For this review, take the finished solid that the model builds, in its own axes (mm). Face numbers are marked on the shaded views. A direction names the side the tool comes from. Give positions to 0.01 mm unless a question says otherwise; leave off trailing zeros. Write each loop counter-clockwise with the first axis right and the second up, starting at its lowest first coordinate (ties: lowest second). Pieces come first, ordered by that corner, then holes. Notation, with made-up numbers: (8.5, 1.25) -> (19.5, 1.25) arc R31 ccw to (19.5, 40.25) -> close; hole circle Ø4 at (59, 65.5). An arc over 180 degrees is marked (long way). Answer as CSV lines item,"result".
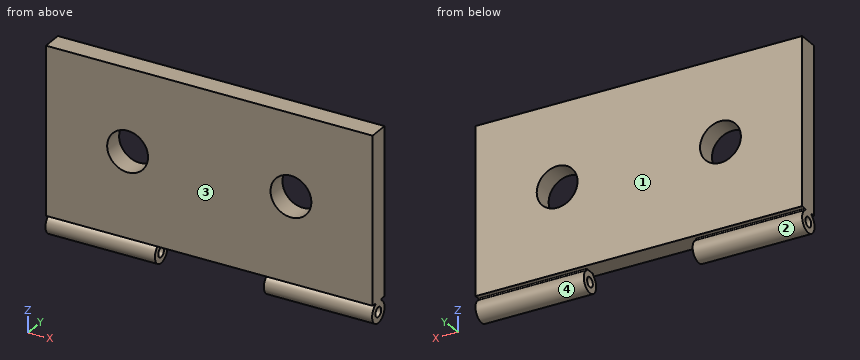
```python
from build123d import *

# Parameters (mm, degrees)
CROQUIS3_W              = 50.8
CROQUIS3_H              = 25.4
CROQUIS3_R              = 3.175
SALIENTE_EXTRUIR1_DEPTH = 3.175
CROQUIS6_R              = 0.762
SALIENTE_EXTRUIR3_DEPTH = 8.466666667
CROQUIS7_R              = 0.762
SALIENTE_EXTRUIR4_DEPTH = 50.8
CROQUIS8_W              = 16.933333333
CROQUIS8_H              = 3.302
CORTAR_EXTRUIR2_DEPTH   = 25.4


with BuildPart() as part:
    # Croquis3 → Saliente-Extruir1 (new body)
    with BuildSketch(Plane(origin=(0, 0, 0), x_dir=(1, 0, 0), z_dir=(0, 1, 0))):
        Rectangle(CROQUIS3_W, CROQUIS3_H)
        with Locations((-12.7, 0)):
            Circle(CROQUIS3_R, mode=Mode.SUBTRACT)
        with Locations((12.7, 0)):
            Circle(CROQUIS3_R, mode=Mode.SUBTRACT)
    extrude(amount=SALIENTE_EXTRUIR1_DEPTH)

    # Croquis6 → Saliente-Extruir3 (add, symmetric)
    with BuildSketch(Plane.ZY):
        with BuildLine():
            Line((-12.7, 3.175), (-13.208, 3.175))
            Line((-13.208, 3.175), (-13.208, 2.437497499))
            ThreePointArc((-13.208, 2.437497499), (-13.301057822, 2.315117237), (-13.443857143, 2.372082497))
            ThreePointArc((-13.443857143, 2.372082497), (-16.51, 1.521687475), (-13.443857143, 0.671292453))
            ThreePointArc((-13.443857143, 0.671292453), (-13.301057822, 0.728257713), (-13.208, 0.605877451))
            Line((-13.208, 0.605877451), (-13.208, 0))
            Line((-13.208, 0), (-12.7, 0))
            Line((-12.7, 0), (-12.7, 3.175))
        make_face()
        with Locations((-14.859, 1.521687475)):
            Circle(CROQUIS6_R, mode=Mode.SUBTRACT)
    extrude(amount=SALIENTE_EXTRUIR3_DEPTH, both=True)

    # Croquis7 → Saliente-Extruir4 (add)
    with BuildSketch(Plane(origin=(25.4, 0, 0), x_dir=(0, 0, -1), z_dir=(1, 0, 0))):
        with BuildLine():
            Line((12.7, 3.175), (13.208, 3.175))
            Line((13.208, 3.175), (13.208, 2.437497499))
            ThreePointArc((13.208, 2.437497499), (13.301057822, 2.315117237), (13.443857143, 2.372082497))
            ThreePointArc((13.443857143, 2.372082497), (16.51, 1.521687475), (13.443857143, 0.671292453))
            ThreePointArc((13.443857143, 0.671292453), (13.301057822, 0.728257713), (13.208, 0.605877451))
            Line((13.208, 0.605877451), (13.208, 0))
            Line((13.208, 0), (12.7, 0))
            Line((12.7, 0), (12.7, 3.175))
        make_face()
        with Locations((14.859, 1.521687475)):
            Circle(CROQUIS7_R, mode=Mode.SUBTRACT)
    extrude(amount=-SALIENTE_EXTRUIR4_DEPTH)

    # Croquis8 → Cortar-Extruir2 (cut)
    with BuildSketch(Plane(origin=(0, 3.175, 0), x_dir=(1, 0, 0), z_dir=(0, 1, 0))):
        with Locations((0.09605237, 14.859)):
            Rectangle(CROQUIS8_W, CROQUIS8_H)
    extrude(amount=-CORTAR_EXTRUIR2_DEPTH, mode=Mode.SUBTRACT)


solid = part.part
```
Q1. For the marked faces 3 and 4, list the 3-axis set-ups (+Z, -Z, +X, -X, +Y, -Y) from which the entire face can be reached by the end or side of a thin tool; tool diameter is ignored.
Answer block:
face 3,"+Z, +X, -X, -Y"
face 4,"+X, -X"
Q2. To check wall thickness, follow probe 1 along X at (y, z) = (1.4, 0) (3 decimals); probe 2 along Z at (x, y) = (10, 0.35); probe 3 along Z at (x, y) = (-13.5, 2.95). State the ranges of each line that lie inside material, in increasing order. Write a range as [from, to].
Answer block:
probe 1,"x = [-25.4, -15.875], [-9.525, 9.525], [15.875, 25.4]"
probe 2,"z = [-16.02, -13.7], [-13.21, -1.67], [1.67, 12.7]"
probe 3,"z = [-15.69, -14.03], [-13.21, -3.07], [3.07, 12.7]"
Q3. Add section B-B (x = 12.7). State how many separate pieces and enclosed holes the cut face has, plus the area to 3 significant figures.
Answer block:
separate pieces,"2"
enclosed holes,"1"
area,"68.9 mm2"
Q4. Add section D-D (z = -6.75). Write out the cut boundary in (x, y) (3 decimals), plus the area to 3 significant figures.
Answer block:
outline,"(-25.4, 0) -> (25.4, 0) -> (25.4, 3.175) -> (-25.4, 3.175) -> close"
area,"161 mm2"
Q5. Add section A-A (z = 0). Write out the cut boundary in (x, y) (3 decimals), plus the area to 3 significant figures.
Answer block:
outline,"(-25.4, 0) -> (-15.875, 0) -> (-15.875, 3.175) -> (-25.4, 3.175) -> close; (-9.525, 0) -> (9.525, 0) -> (9.525, 3.175) -> (-9.525, 3.175) -> close; (15.875, 0) -> (25.4, 0) -> (25.4, 3.175) -> (15.875, 3.175) -> close"
area,"121 mm2"
Q6. Draft analysis for pull direction Z (two halves, no side actions). For the marked faces 1 and 2, state which applies: released by +Z, released by -Z, zero draft, split by the parting line, or undercut.
Answer block:
face 1,"zero draft"
face 2,"undercut"
Q7. Clearance check with flat-ended pins moving along their axes: pin 1 (2 mm diameter, centred on x = 15, z = 3.5, fed in from -Y); pin 2 (1.2 mm diameter, centred on y = 1.52, z = -14.86, fed in from -X) (1 decimal). State where each tip first meets the part, or that it passes through.
Answer block:
pin 1,"stops at y = 0"
pin 2,"passes through"
